from build123d import *

# Parameters (mm, degrees)
SKETCH2_W           = 32
SKETCH2_H           = 25
SKETCH2_R           = 11
BOSS_EXTRUDE1_DEPTH = 3
SKETCH3_R           = 11
BOSS_EXTRUDE2_DEPTH = 1
SKETCH4_W           = 6
SKETCH4_H           = 3
SKETCH4_W_2         = 3
SKETCH4_H_2         = 6
BOSS_EXTRUDE3_DEPTH = 3


with BuildPart() as part:
    # Sketch2 → Boss-Extrude1 (new body)
    with BuildSketch(Plane.XY):
        Rectangle(SKETCH2_W, SKETCH2_H)
        Circle(SKETCH2_R, mode=Mode.SUBTRACT)
    extrude(amount=BOSS_EXTRUDE1_DEPTH)

    # Sketch3 → Boss-Extrude2 (add)
    with BuildSketch(Plane(origin=(0, 0, 0), x_dir=(-1, 0, 0), z_dir=(0, 0, -1))):
        Circle(SKETCH3_R)
    extrude(amount=-BOSS_EXTRUDE2_DEPTH)

    # Sketch4 → Boss-Extrude3 (add)
    with BuildSketch(Plane(origin=(0, 0, 0), x_dir=(-1, 0, 0), z_dir=(0, 0, -1))):
        with Locations((-13, -14)):
            Rectangle(SKETCH4_W, SKETCH4_H)
        with Locations((-17.5, -9.5)):
            Rectangle(SKETCH4_W_2, SKETCH4_H_2)
        with Locations((-17.5, 0)):
            Rectangle(SKETCH4_W_2, SKETCH4_H_2)
        with Locations((-17.5, 9.5)):
            Rectangle(SKETCH4_W_2, SKETCH4_H_2)
        with Locations((0, 14)):
            Rectangle(SKETCH4_W, SKETCH4_H)
        with Locations((13, 14)):
            Rectangle(SKETCH4_W, SKETCH4_H)
        with Locations((17.5, 9.5)):
            Rectangle(SKETCH4_W_2, SKETCH4_H_2)
        with Locations((17.5, 0)):
            Rectangle(SKETCH4_W_2, SKETCH4_H_2)
        with Locations((17.5, -9.5)):
            Rectangle(SKETCH4_W_2, SKETCH4_H_2)
        with Locations((13, -14)):
            Rectangle(SKETCH4_W, SKETCH4_H)
        with Locations((0, -14)):
            Rectangle(SKETCH4_W, SKETCH4_H)
        with Locations((-13, 14)):
            Rectangle(SKETCH4_W, SKETCH4_H)
    extrude(amount=-BOSS_EXTRUDE3_DEPTH)


solid = part.part
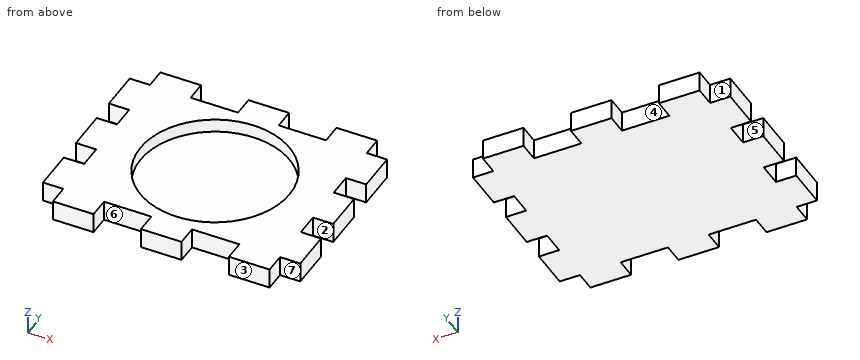
Could you check a few things on this model? Use its own coordinates, in mm. Face numbers are marked on the shaded views. A direction names the side the tool comes from. Give positions to 0.01 mm unless a question says otherwise; leave off trailing zeros. Write each loop counter-clockwise with the first axis right and the second up, starting at its lowest first coordinate (ties: lowest second). Pieces come first, ordered by that corner, then holes. Notation, with made-up numbers: (19, 23) -> (39, 23) arc R30 ccw to (39, 46) -> close; hole circle Ø11 at (22, -23). An arc over 180 degrees is marked (long way). Answer as a JSON object with one key per item and string values.
Q1. Which directions (+Z, -Z, +X, -X, +Y, -Y) give clear straight access to the entire face, cutting with the end or side of a thin tool? Please do the marked faces 4, 5, 6 and 7.
Taken from the geometry:
{"face 4": "+Z, -Z, +Y", "face 5": "+Z, -Z, -X", "face 6": "+Z, -Z, -Y", "face 7": "+Z, -Z, +X, -Y"}
Q2. We'd pull the mould along Y, two halves only. Please class the marked faces 1, 2 and 3: released by +Y, released by -Y, zero draft, split by the parting line, or undercut.
Taken from the geometry:
{"face 1": "released by +Y", "face 2": "undercut", "face 3": "released by -Y"}
Q3. Please list where these lines run through material, in increasing order: L1, parallel to X at y = -13, z = 2.1; L2, parallel to X at y = 0, z = 2.1; L3, parallel to Y at x = 0, z = 2.6.
Taken from the geometry:
{"L1": "x = -16 to -10, -3 to 3, 10 to 16", "L2": "x = -19 to -11, 11 to 19", "L3": "y = -15.5 to -11, 11 to 15.5"}
Q4. Suppose I cut it at A-A on y = 0. Write out the boundary of the cut face in (x, z).
Taken from the geometry:
{"outline": "(-19, 0) -> (19, 0) -> (19, 3) -> (11, 3) -> (11, 1) -> (-11, 1) -> (-11, 3) -> (-19, 3) -> close"}
Q5. Will these pins go through, and if not, where does the flat tip stop? pin 1 Ø1.5 at (y, z) = (13.5, 2) entering from +X; pin 2 Ø1.5 at (x, y) = (-1.5, -2) entering from +Z; pin 3 Ø1.5 at (y, z) = (4.5, 1.5) entering from -X.
Taken from the geometry:
{"pin 1": "stops at x = 16", "pin 2": "stops at z = 1", "pin 3": "stops at x = -16"}
Q6. Suppose I cut it at B-B on x = 0. Write out the boundary of the cut face in (y, z), then the cut area to 3 significant figures.
Taken from the geometry:
{"outline": "(-15.5, 0) -> (15.5, 0) -> (15.5, 3) -> (11, 3) -> (11, 1) -> (-11, 1) -> (-11, 3) -> (-15.5, 3) -> close", "area": "49.0 mm²"}
